```python
from build123d import *

# Parameters (mm, degrees)
SKETCH1_R           = 2.45
SKETCH1_R_2         = 2.05
BOSS_EXTRUDE1_DEPTH = 24
CUT_EXTRUDE1_START  = 9
SKETCH1_4_R         = 2.45
CUT_EXTRUDE1_DEPTH  = 6
SKETCH1_5_R         = 2.45
CUT_EXTRUDE3_DEPTH  = 44
FILLET1_R           = 3


with BuildPart() as part:
    # Sketch1 → Boss-Extrude1 (new body)
    # profile 1 of 7: a face of its own
    with BuildSketch(Plane.XY):
        with BuildLine():
            ThreePointArc((-20.35, 15.35), (-18.885533906, 18.885533906), (-15.35, 20.35))
            Line((-15.35, 20.35), (15.35, 20.35))
            ThreePointArc((15.35, 20.35), (18.885533906, 18.885533906), (20.35, 15.35))
            Line((20.35, 15.35), (20.35, -15.35))
            ThreePointArc((20.35, -15.35), (18.885533906, -18.885533906), (15.35, -20.35))
            Line((15.35, -20.35), (-15.35, -20.35))
            ThreePointArc((-15.35, -20.35), (-18.885533906, -18.885533906), (-20.35, -15.35))
            Line((-20.35, -15.35), (-20.35, 15.35))
        make_face()
        with Locations((0, -15.5)):
            Circle(SKETCH1_R, mode=Mode.SUBTRACT)
        with Locations((15.5, 14.200476627)):
            Circle(SKETCH1_R, mode=Mode.SUBTRACT)
        with Locations((-15.5, 14.200476627)):
            Circle(SKETCH1_R, mode=Mode.SUBTRACT)
        Circle(SKETCH1_R_2, mode=Mode.SUBTRACT)
    # profile 2 of 7: a face of its own
    with BuildSketch(Plane.XY):
        with BuildLine():
            Line((-20.35, 15.35), (-20.35, 4.327407195))
            ThreePointArc((-20.35, 4.327407195), (-9.684073591, 4.863721302), (-4.5, 14.200476627))
            ThreePointArc((-4.5, 14.200476627), (-4.980365863, 17.415643439), (-6.37950866, 20.35))
            Line((-6.37950866, 20.35), (-15.35, 20.35))
            ThreePointArc((-15.35, 20.35), (-18.885533906, 18.885533906), (-20.35, 15.35))
        make_face()
        with Locations((-15.5, 14.200476627)):
            Circle(SKETCH1_R, mode=Mode.SUBTRACT)
    # profile 3 of 7: a face of its own
    with BuildSketch(Plane.XY):
        with Locations((-15.5, 14.200476627)):
            Circle(SKETCH1_R)
    # profile 4 of 7: a face of its own
    with BuildSketch(Plane.XY):
        with BuildLine():
            ThreePointArc((11, -15.5), (-2.489602002, -4.785435992), (-9.873069432, -20.35))
            Line((-9.873069432, -20.35), (9.873069432, -20.35))
            ThreePointArc((9.873069432, -20.35), (10.714564008, -17.989602002), (11, -15.5))
        make_face()
        with Locations((0, -15.5)):
            Circle(SKETCH1_R, mode=Mode.SUBTRACT)
    # profile 5 of 7: a face of its own
    with BuildSketch(Plane.XY):
        with Locations((0, -15.5)):
            Circle(SKETCH1_R)
    # profile 6 of 7: a face of its own
    with BuildSketch(Plane.XY):
        with BuildLine():
            Line((15.35, 20.35), (6.37950866, 20.35))
            ThreePointArc((6.37950866, 20.35), (7.209032378, 6.971378766), (20.35, 4.327407195))
            Line((20.35, 4.327407195), (20.35, 15.35))
            ThreePointArc((20.35, 15.35), (18.885533906, 18.885533906), (15.35, 20.35))
        make_face()
        with Locations((15.5, 14.200476627)):
            Circle(SKETCH1_R, mode=Mode.SUBTRACT)
    # profile 7 of 7: a face of its own
    with BuildSketch(Plane.XY):
        with Locations((15.5, 14.200476627)):
            Circle(SKETCH1_R)
    extrude(amount=BOSS_EXTRUDE1_DEPTH)

    # Sketch1_4 → Cut-Extrude1 (cut)
    # profile 1 of 9: a face of its own
    with BuildSketch(Plane.XY.offset(CUT_EXTRUDE1_START)):
        with BuildLine():
            ThreePointArc((-6.37950866, 20.35), (-23.790967622, 21.429574488), (-20.35, 4.327407195))
            Line((-20.35, 4.327407195), (-20.35, 15.35))
            ThreePointArc((-20.35, 15.35), (-18.885533906, 18.885533906), (-15.35, 20.35))
            Line((-15.35, 20.35), (-6.37950866, 20.35))
        make_face()
    # profile 2 of 9: a face of its own
    with BuildSketch(Plane.XY.offset(CUT_EXTRUDE1_START)):
        with BuildLine():
            Line((-20.35, 15.35), (-20.35, 4.327407195))
            ThreePointArc((-20.35, 4.327407195), (-9.684073591, 4.863721302), (-4.5, 14.200476627))
            ThreePointArc((-4.5, 14.200476627), (-4.980365863, 17.415643439), (-6.37950866, 20.35))
            Line((-6.37950866, 20.35), (-15.35, 20.35))
            ThreePointArc((-15.35, 20.35), (-18.885533906, 18.885533906), (-20.35, 15.35))
        make_face()
        with Locations((-15.5, 14.200476627)):
            Circle(SKETCH1_4_R, mode=Mode.SUBTRACT)
    # profile 3 of 9: a face of its own
    with BuildSketch(Plane.XY.offset(CUT_EXTRUDE1_START)):
        with Locations((-15.5, 14.200476627)):
            Circle(SKETCH1_4_R)
    # profile 4 of 9: a face of its own
    with BuildSketch(Plane.XY.offset(CUT_EXTRUDE1_START)):
        with BuildLine():
            Line((15.35, 20.35), (6.37950866, 20.35))
            ThreePointArc((6.37950866, 20.35), (7.209032378, 6.971378766), (20.35, 4.327407195))
            Line((20.35, 4.327407195), (20.35, 15.35))
            ThreePointArc((20.35, 15.35), (18.885533906, 18.885533906), (15.35, 20.35))
        make_face()
        with Locations((15.5, 14.200476627)):
            Circle(SKETCH1_4_R, mode=Mode.SUBTRACT)
    # profile 5 of 9: a face of its own
    with BuildSketch(Plane.XY.offset(CUT_EXTRUDE1_START)):
        with Locations((15.5, 14.200476627)):
            Circle(SKETCH1_4_R)
    # profile 6 of 9: a face of its own
    with BuildSketch(Plane.XY.offset(CUT_EXTRUDE1_START)):
        with BuildLine():
            ThreePointArc((26.5, 14.200476627), (18.715166812, 24.720110764), (6.37950866, 20.35))
            Line((6.37950866, 20.35), (15.35, 20.35))
            ThreePointArc((15.35, 20.35), (18.885533906, 18.885533906), (20.35, 15.35))
            Line((20.35, 15.35), (20.35, 4.327407195))
            ThreePointArc((20.35, 4.327407195), (24.836755325, 8.384550218), (26.5, 14.200476627))
        make_face()
    # profile 7 of 9: a face of its own
    with BuildSketch(Plane.XY.offset(CUT_EXTRUDE1_START)):
        with BuildLine():
            ThreePointArc((11, -15.5), (-2.489602002, -4.785435992), (-9.873069432, -20.35))
            Line((-9.873069432, -20.35), (9.873069432, -20.35))
            ThreePointArc((9.873069432, -20.35), (10.714564008, -17.989602002), (11, -15.5))
        make_face()
        with Locations((0, -15.5)):
            Circle(SKETCH1_4_R, mode=Mode.SUBTRACT)
    # profile 8 of 9: a face of its own
    with BuildSketch(Plane.XY.offset(CUT_EXTRUDE1_START)):
        with Locations((0, -15.5)):
            Circle(SKETCH1_4_R)
    # profile 9 of 9: a face of its own
    with BuildSketch(Plane.XY.offset(CUT_EXTRUDE1_START)):
        with BuildLine():
            Line((9.873069432, -20.35), (-9.873069432, -20.35))
            ThreePointArc((-9.873069432, -20.35), (0, -26.5), (9.873069432, -20.35))
        make_face()
    extrude(amount=CUT_EXTRUDE1_DEPTH, mode=Mode.SUBTRACT)

    # Sketch1_5 → Cut-Extrude3 (cut)
    with BuildSketch(Plane.XY):
        with Locations((-15.5, 14.200476627)):
            Circle(SKETCH1_5_R)
        with Locations((0, -15.5)):
            Circle(SKETCH1_5_R)
        with Locations((15.5, 14.200476627)):
            Circle(SKETCH1_5_R)
    extrude(amount=CUT_EXTRUDE3_DEPTH, mode=Mode.SUBTRACT)

    # Fillet1
    fillet1_edges = [part.edges().sort_by_distance(p)[0] for p in [
        (20.35, 4.327407195, 12),
        (9.873069432, -20.35, 12),
        (-9.873069432, -20.35, 12),
        (-20.35, 4.327407195, 12),
        (6.37950866, 20.35, 12),
        (-6.37950866, 20.35, 12),
    ]]
    fillet(fillet1_edges, radius=FILLET1_R)


solid = part.part
```
Geometry: final body of the model. Coordinates: model frame, mm. Round coordinates to 2 decimals unless told otherwise and drop trailing zeros. Order: outer loops, then holes, each group sorted by start corner. A loop starts at its lowest first (then second) coordinate and runs counter-clockwise, first axis right, second up. Notation, with made-up numbers: M 14,3.5 L 68,3.5 A25 ccw 68,30.5 Z; hole C 89.25,25 d2. An arc over 180 degrees is marked long. Use one line per item in the form item = value. Start each with the question number.
Q1. Material intervals for line 1 (Y direction, x = 0, z = 6.75); line 2 (Y direction, x = 0, z = 11); line 3 (Y direction, x = -15.5, z = 17.25), sorted ascending. Write a range as [from, to].
Q2. Cut plane D-D (x = -7). Return loops of the section in (y, z), and give its area (3 significant figures).
Q3. Cut plane C-C (y = -6.5). Return loops of the section in (x, z), and give its area (3 significant figures).
Q4. Cut plane B-B (z = 15.5). Return loops of the section in (x, y), and give its area (3 significant figures).
Q5. Mould query, pull axis X, two halves, no side actions, for faces 1 (the face through (-11.64, -19.35, 12.04)), 2 (the face through (20.35, 0, 12)), 3 (the face through (-18.92, 18.85, 4.44)), 4 (the face through (-17.444, 12.71, 4.437)). Classes: +X half, -X half, draft (parallel to the pull), parting line (faces both ways), or undercut.
Q6. Cut plane A-A (x = 0). Return loops of the section in (y, z), and give its area (3 significant figures).
Q7. Pin query (flat end, axial travel): pin 1 Ø10 at (x, y) = (-14, -15.5) entering from -Z; pin 2 Ø4.5 at (x, y) = (15.5, 14.2) entering from +Z. Return the tip coordinate at first contact, or that it passes through.
Geometry results:
q1.line_1 = [-20.35, -17.95], [-13.05, -2.05], [2.05, 20.35]
q1.line_2 = [-4.5, -2.05], [2.05, 20.35]
q1.line_3 = [-20.35, 11.75], [16.65, 20.35]
q2.outline = M -20.35,0 L 20.35,0 L 20.35,9 L 7.22,9 L 7.22,15 L 20.35,15 L 20.35,24 L -20.35,24 L -20.35,15 L -7.01,15 L -7.01,9 L -20.35,9 Z
q2.area = 818 mm^2
q3.outline = M -20.35,0 L 20.35,0 L 20.35,24 L -20.35,24 Z; hole M -6.32,9 L 6.32,9 L 6.32,15 L -6.32,15 Z
q3.area = 901 mm^2
q4.outline = M -20.35,-15.35 A5 ccw -15.35,-20.35 L 15.35,-20.35 A5 ccw 20.35,-15.35 L 20.35,15.35 A5 ccw 15.35,20.35 L -15.35,20.35 A5 ccw -20.35,15.35 Z; hole C -15.5,14.2 d4.9; hole C 0,-15.5 d4.9; hole C 0,0 d4.1; hole C 15.5,14.2 d4.9
q4.area = 1,570 mm^2
q5.face_1 = undercut
q5.face_2 = +X half
q5.face_3 = -X half
q5.face_4 = undercut
q6.outline = M -20.35,0 L -17.95,0 L -17.95,9 L -20.35,9 Z; M -20.35,15 L -17.95,15 L -17.95,24 L -20.35,24 Z; M -13.05,0 L -2.05,0 L -2.05,24 L -13.05,24 L -13.05,15 L -4.5,15 L -4.5,9 L -13.05,9 Z; M 2.05,0 L 20.35,0 L 20.35,24 L 2.05,24 Z
q6.area = 695 mm^2
q7.pin_1 = 0
q7.pin_2 = through
